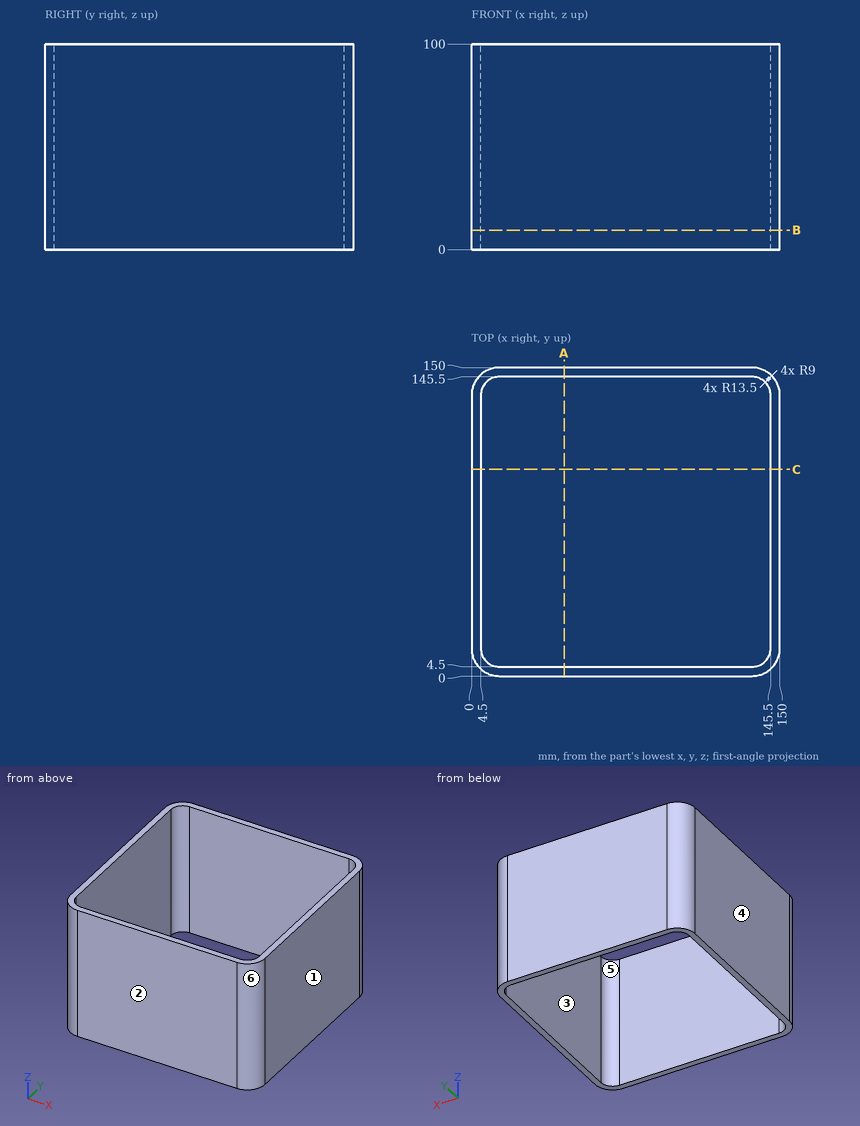
Drawing for the job (mm, zero at the part's lowest x, y, z). A direction names the side the tool comes from. Coordinates: 2 decimals unless noted, no trailing zeros. Order: outer loops, then holes, each group sorted by start corner. A loop starts at its lowest first (then second) coordinate and runs counter-clockwise, first axis right, second up. Notation, with made-up numbers: (44, 38.25) -> (78, 38.25) arc R10 ccw to (78, 48.25) -> close; hole circle Ø4 at (29.25, 67.5). An arc over 180 degrees is marked (long way). Return JSON: item names as keys, results as strings.
Item 1: Slice it at B-B (z = 9.5). Write the cut outline in (x, y), then the cut area to 3 significant figures.
Model answer:
{"outline": "(0, 13.5) arc R13.5 ccw to (13.5, 0) -> (136.5, 0) arc R13.5 ccw to (150, 13.5) -> (150, 136.5) arc R13.5 ccw to (136.5, 150) -> (13.5, 150) arc R13.5 ccw to (0, 136.5) -> close; hole (4.5, 13.5) arc R9 ccw to (13.5, 4.5) -> (136.5, 4.5) arc R9 ccw to (145.5, 13.5) -> (145.5, 136.5) arc R9 ccw to (136.5, 145.5) -> (13.5, 145.5) arc R9 ccw to (4.5, 136.5) -> close", "area": "2,530 mm²"}
Item 2: Wall check: line 1 along Y through (x, z) = (81, 18); line 2 along Y through (x, z) = (8, 34). Give the ranges that are in metal, low to high. Write a range as from..to.
Model answer:
{"line 1": "y = 0..4.5, 145.5..150", "line 2": "y = 1.17..6.38, 143.62..148.83"}
Item 3: 3-axis set-ups, long thin cutter, end or side, ignore diameter. For the marked faces 5 and 6: which of +Z, -Z, +X, -X, +Y, -Y reach the whole face in a straight line?
Model answer:
{"face 5": "+Z, -Z", "face 6": "+Z, -Z, +X, -Y"}
Item 4: Pin check, flat tip, straight feed: P1, Ø3, axis at x = 46.5, z = 28.5, coming from the -Y side. Stop position of the tip, or through.
Model answer:
{"P1": "stops at y = 0"}
Item 5: Slice it at A-A (x = 45). Write the cut outline in (y, z), then the cut area to 3 significant figures.
Model answer:
{"outline": "(0, 0) -> (4.5, 0) -> (4.5, 100) -> (0, 100) -> close; (145.5, 0) -> (150, 0) -> (150, 100) -> (145.5, 100) -> close", "area": "900 mm²"}
Item 6: Mould opens along X. For the marked faces 1, 2, 3 and 4 say: pulls with the +X half, pulls with the -X half, needs draft (parallel to the pull), parting line crosses it, or undercut.
Model answer:
{"face 1": "pulls with the +X half", "face 2": "needs draft", "face 3": "undercut", "face 4": "pulls with the -X half"}
